Geometry: final body of the model. Coordinates: model frame, mm. Give positions to 0.01 mm unless a question says otherwise; leave off trailing zeros. Order: outer loops, then holes, each group sorted by start corner. A loop starts at its lowest first (then second) coordinate and runs counter-clockwise, first axis right, second up. Notation, with made-up numbers: (-20.75, -34.5) - (17.25, -34.5) arc R31 ccw to (17.25, -9.5) - close; hole circle Ø3 at (13.5, -6). An arc over 180 degrees is marked (long way). Use one line per item in the form item = value.
Autodesk Inventor part; units mm, degrees
ref_plane "YZ Plane" through (0, 0, 0) normal (1, 0, 0) x (0, 1, 0)
ref_plane "XZ Plane" through (0, 0, 0) normal (0, 1, 0) x (-1, 0, 0)
ref_plane "XY Plane" through (0, 0, 0) normal (0, 0, 1) x (1, 0, 0)
sketch "Sketch1" plane through (0, 0, 0) normal (0, 1, 0) x (-1, 0, 0)
  line L0 (-175, 175) -> (-175, -175)
  line L1 (-175, -175) -> (175, -175)
  line L2 (175, -175) -> (175, 175)
  line L3 (175, 175) -> (-175, 175)
  line L4 (-175, 175) -> (175, -175) construction
  line L5 (-175, -175) -> (175, 175) construction
  line L6 (-86.5, 86.5) -> (86.5, 86.5)
  line L7 (86.5, 86.5) -> (86.5, -86.5)
  line L8 (86.5, -86.5) -> (-86.5, -86.5)
  line L9 (-86.5, -86.5) -> (-86.5, 86.5)
  line L10 (-86.5, 86.5) -> (86.5, -86.5) construction
  line L11 (86.5, 86.5) -> (-86.5, -86.5) construction
  line L12 (-66.5, 66.5) -> (-66.5, -66.5)
  line L13 (-66.5, -66.5) -> (66.5, -66.5)
  line L14 (66.5, -66.5) -> (66.5, 66.5)
  line L15 (66.5, 66.5) -> (-66.5, 66.5)
  line L16 (-66.5, 66.5) -> (66.5, -66.5) construction
  line L17 (-66.5, -66.5) -> (66.5, 66.5) construction
  line L18 (86.5, 0) -> (86.5, 20)
  line L19 (0, 233.3952) -> (0, -224.0457) construction
  line L20 (-86.5, -66.5) -> (-76.5, -66.5)
  line L21 (-76.5, -66.5) -> (-76.5, -76.5)
  line L22 (-76.5, -76.5) -> (-66.5, -76.5)
  line L23 (-66.5, -76.5) -> (-66.5, -86.5)
  line L24 (-66.5, 86.5) -> (-86.5, 86.5) construction
  line L25 (-86.5, 86.5) -> (-86.5, 66.5) construction
  line L26 (-86.5, 20) -> (-86.5, -20) construction
  line L27 (-86.5, -66.5) -> (-86.5, -86.5) construction
  line L28 (-86.5, -86.5) -> (-66.5, -86.5) construction
  point P0 (0, 0)
  dimension "d0" = 350
  dimension "d1" = 350
  dimension "d2" = 173
  dimension "d3" = 173
  dimension "d4" = 133
  dimension "d5" = 133
extrude "Extrusion1" add sketch "Sketch1" along normal blind 6.35 contours L3 L2 L1 L0 | L6 L7 L8 L23 L22 L21 L20 L9 | L20 L21 L22 L23 L8 L9
sketch "Sketch2" plane through (0, 6.35, 0) normal (0, 1, 0) x (1, 0, 0)
  line L0 (86.5, -86.5) -> (86.5, 86.5)
  line L1 (86.5, 86.5) -> (-86.5, 86.5)
  line L2 (-86.5, 86.5) -> (-86.5, -86.5)
  line L3 (-86.5, -86.5) -> (86.5, -86.5)
  line L4 (86.5, -86.5) -> (-86.5, 86.5) construction
  line L5 (86.5, 86.5) -> (-86.5, -86.5) construction
  line L6 (-66.5, -86.5) -> (-66.5, -76.5)
  line L7 (-66.5, -76.5) -> (-76.5, -76.5)
  line L8 (-76.5, -76.5) -> (-76.5, -66.5)
  line L9 (-76.5, -66.5) -> (-86.5, -66.5)
  line L10 (-86.5, -66.5) -> (-86.5, -86.5)
  line L11 (-86.5, -86.5) -> (-66.5, -86.5)
  line L12 (-86.5, 0) -> (-86.5, -20)
  line L13 (-86.5, -20) -> (-76.5, -20)
  line L14 (-76.5, -20) -> (-76.5, 20)
  line L15 (-76.5, 20) -> (-86.5, 20)
  line L16 (-86.5, 20) -> (-86.5, 0)
  line L17 (-66.5, 86.5) -> (-66.5, 76.5)
  line L18 (-66.5, 76.5) -> (-76.5, 76.5)
  line L19 (-76.5, 76.5) -> (-76.5, 66.5)
  line L20 (-76.5, 66.5) -> (-86.5, 66.5)
  line L21 (0, -182.5609) -> (0, 182.5037) construction
  line L22 (66.5, -86.5) -> (66.5, -76.5)
  line L23 (66.5, -76.5) -> (76.5, -76.5)
  line L24 (76.5, -76.5) -> (76.5, -66.5)
  line L25 (76.5, -66.5) -> (86.5, -66.5)
  line L26 (86.5, -20) -> (76.5, -20)
  line L27 (76.5, -20) -> (76.5, 20)
  line L28 (76.5, 20) -> (86.5, 20)
  line L29 (66.5, 86.5) -> (66.5, 76.5)
  line L30 (66.5, 76.5) -> (76.5, 76.5)
  line L31 (76.5, 76.5) -> (76.5, 66.5)
  line L32 (76.5, 66.5) -> (86.5, 66.5)
  point P0 (0, 0)
  dimension "d17" = 173
  dimension "d18" = 173
  dimension "d19" = 10
  dimension "d20" = 10
  dimension "d21" = 10
  dimension "d22" = 20
  dimension "d23" = 10
  dimension "d24" = 40
  dimension "d25" = 10
  dimension "d26" = 10
  dimension "d27" = 10
  dimension "d28" = 10
extrude "Extrusion2" cut sketch "Sketch2" against normal blind 6.35 contours L3 L2 L9 L8 L7 L6 | L2 L15 L14 L13 | L17 L18 L19 L20 L2 L1
ref_plane "Work Plane1" through (0, 0, 175) normal (1, 0, 0) x (0, 0, -1)
mirror "Mirror1" about plane through (0, 0, 175) normal (1, 0, 0) of "Extrusion2"
ref_plane "Work Plane2" through (0, 0, 175) normal (1, 0, 0) x (0, 0, -1)
properties part number "Milestone 2 Main Vehicle Chassis"
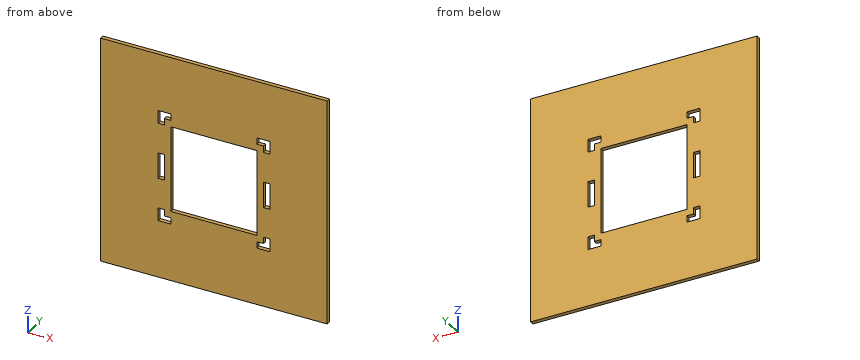
(1) Ray query, line 1 along X through (y, z) = (3.75, -9); line 2 along X through (y, z) = (5.5, -79); line 3 along X through (y, z) = (4.25, 68). Return the intervals inside material, ascending.
Computed values:
line_1 = -175 to -86.5, -76.5 to -66.5, 66.5 to 76.5, 86.5 to 175
line_2 = -175 to -86.5, -66.5 to 66.5, 86.5 to 175
line_3 = -175 to -86.5, -76.5 to 76.5, 86.5 to 175
(2) Cut plane D-D on y = 3.5. Give the number of separate pieces and of enclosed holes in the cut face, plus the area to 3 significant figures.
Computed values:
separate_pieces = 1
enclosed_holes = 7
area = 103,000 mm²
(3) Cut plane B-B on x = -33. Output: boundary loops of the cut face in (y, z), plus the area to 3 significant figures.
Computed values:
outline = (0, -175) - (6.35, -175) - (6.35, -66.5) - (0, -66.5) - close; (0, 66.5) - (6.35, 66.5) - (6.35, 175) - (0, 175) - close
area = 1,380 mm²
(4) Cut plane A-A on z = -12. Output: boundary loops of the cut face in (x, y).
Computed values:
outline = (-175, 0) - (-86.5, 0) - (-86.5, 6.35) - (-175, 6.35) - close; (-76.5, 0) - (-66.5, 0) - (-66.5, 6.35) - (-76.5, 6.35) - close; (66.5, 0) - (76.5, 0) - (76.5, 6.35) - (66.5, 6.35) - close; (86.5, 0) - (175, 0) - (175, 6.35) - (86.5, 6.35) - close
(5) Cut plane C-C on z = 31. Output: boundary loops of the cut face in (x, y), plus the area to 3 significant figures.
Computed values:
outline = (-175, 0) - (-66.5, 0) - (-66.5, 6.35) - (-175, 6.35) - close; (66.5, 0) - (175, 0) - (175, 6.35) - (66.5, 6.35) - close
area = 1,380 mm²
